Can you work these out from the drawing? Everything is in mm from the part's minimum corner. A direction names the side the tool comes from. Give positions to 0.01 mm unless a question says otherwise; leave off trailing zeros. Write each loop counter-clockwise with the first axis right and the second up, starting at its lowest first coordinate (ties: lowest second). Pieces come first, ordered by that corner, then holes. Notation, with made-up numbers: (86.25, -8) -> (142.25, -8) arc R17 cw to (142.25, -1) -> close; hole circle Ø3 at (-9, 88.25). An arc over 180 degrees is marked (long way). Return JSON: item names as keys, results as strings.
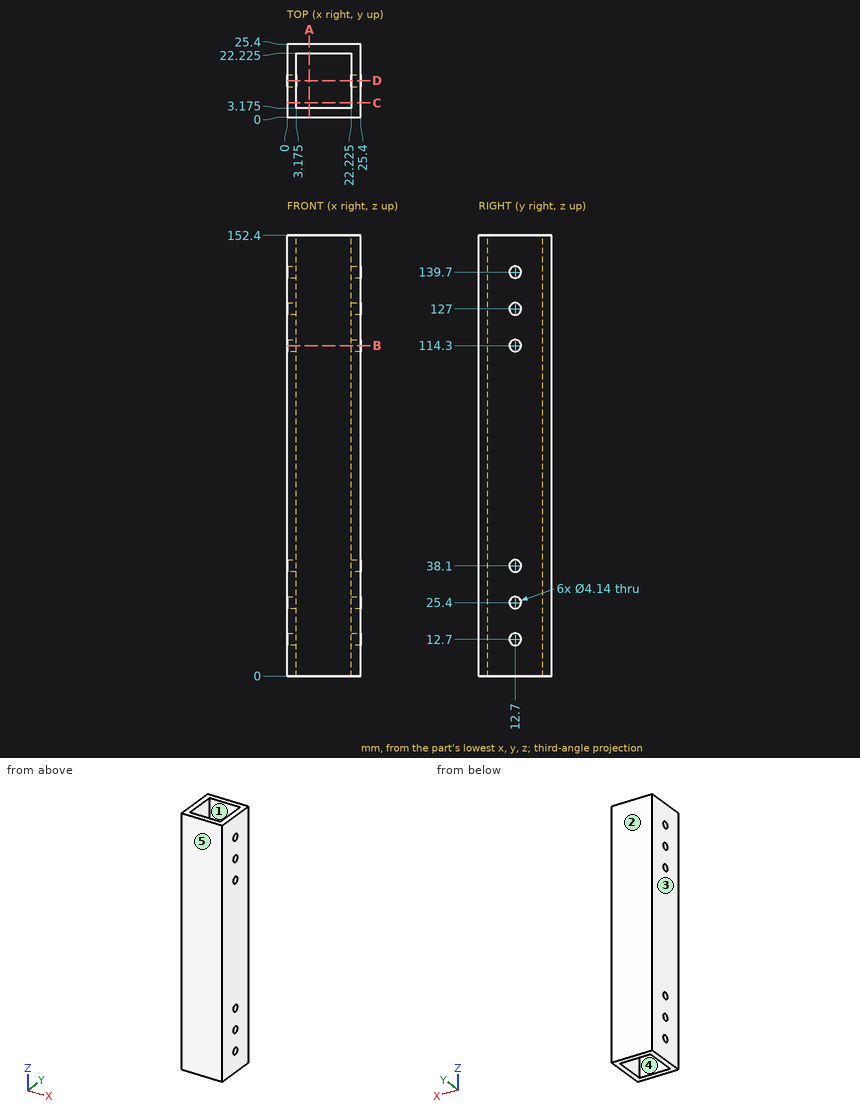
1. Which directions (+Z, -Z, +X, -X, +Y, -Y) give clear straight access to the entire face, cutting with the end or side of a thin tool? Please do the marked faces 1 and 2.
Taken from the geometry:
{"face 1": "+Z, -Z", "face 2": "+Z, -Z, +X, -X, +Y"}
2. If we mould it in two halves opening along X, with no side actions, what happens to the marked faces 3, 4 and 5? For each: released by +X, released by -X, zero draft, split by the parting line, or undercut.
Taken from the geometry:
{"face 3": "released by -X", "face 4": "undercut", "face 5": "zero draft"}
3. For pin 1 Ø5 at (x, y) = (7, 18) entering from +Z; pin 2 Ø5.5 at (y, z) = (12.7, 25.4) entering from +X, each with a flat end and sliding along its axis, tell me the tip position at first contact or that it passes through.
Taken from the geometry:
{"pin 1": "passes through", "pin 2": "stops at x = 25.4"}
4. Suppose I cut it at D-D, the plane y = 12.7. Count the separate pieces of the cut face and the enclosed holes in it, and give its area (3 significant figures).
Taken from the geometry:
{"separate pieces": "14", "enclosed holes": "0", "area": "810 mm²"}
5. Suppose I cut it at A-A, the plane x = 7.75. List the corners of the cut face in (y, z) for me (3 decimals).
Taken from the geometry:
{"outline": "(0, 0) -> (3.175, 0) -> (3.175, 152.4) -> (0, 152.4) -> close; (22.225, 0) -> (25.4, 0) -> (25.4, 152.4) -> (22.225, 152.4) -> close"}
6. If I drill on line 1 (Y direction, x = 5.25, z = 115) (3 decimals); line 2 (Y direction, x = 23.9, z = 139.7), over which ranges is the centre line in solid material (lowest first)? Write a range as [from, to].
Taken from the geometry:
{"line 1": "y = [0, 3.175], [22.225, 25.4]", "line 2": "y = [0, 10.63], [14.77, 25.4]"}
7. Suppose I cut it at B-B, the plane z = 114.3. List the corners of the cut face in (x, y) for me (1 decimal).
Taken from the geometry:
{"outline": "(0, 0) -> (25.4, 0) -> (25.4, 10.6) -> (22.2, 10.6) -> (22.2, 3.2) -> (3.2, 3.2) -> (3.2, 10.6) -> (0, 10.6) -> close; (0, 14.8) -> (3.2, 14.8) -> (3.2, 22.2) -> (22.2, 22.2) -> (22.2, 14.8) -> (25.4, 14.8) -> (25.4, 25.4) -> (0, 25.4) -> close"}
